from build123d import *

# Parameters (mm, degrees)
BOSS_EXTRU_1_DEPTH       = 68.5
BOSS_EXTRU_2_DEPTH       = 2.5
ESQUISSE4_W              = 95
ESQUISSE4_H              = 54.5
ENL_V_MAT_EXTRU_1_DEPTH  = 2.5
ESQUISSE5_W              = 16
ESQUISSE5_H              = 52.4
ENL_V_MAT_EXTRU_2_DEPTH  = 2.5
BOSS_EXTRU_3_DEPTH       = 2.5
CHANFREIN1_SIZE          = 2.5
CONG_1_R                 = 1.5
ENL_V_MAT_EXTRU_3_DEPTH  = 1.2
CHANFREIN2_SIZE          = 0.3
ESQUISSE8_W              = 20
ESQUISSE8_H              = 1
ENL_V_MAT_EXTRU_4_DEPTH  = 3
CHANFREIN3_SIZE          = 0.5
CHANFREIN4_SIZE          = 0.5
ESQUISSE9_R              = 1
ENL_V_MAT_EXTRU_5_DEPTH  = 75
CHANFREIN5_SIZE          = 1
CHANFREIN6_SIZE          = 1
ENL_V_MAT_EXTRU_6_DEPTH  = 1
ENL_V_START              = -1
ENL_V_MAT_EXTRU_7_DEPTH  = 1
ESQUISSE13_W             = 12
ESQUISSE13_H             = 8
ENL_V_MAT_EXTRU_8_DEPTH  = 2.5
CONG_2_R                 = 1
CHANFREIN7_SIZE          = 0.5
ESQUISSE14_W             = 25.2
ESQUISSE14_H             = 25.2
ENL_V_MAT_EXTRU_9_DEPTH  = 1.45
CHANFREIN8_SIZE          = 0.2
ESQUISSE15_R             = 10.1
ENL_V_MAT_EXTRU_10_DEPTH = 1.05
CHANFREIN9_SIZE          = 0.6


with BuildPart() as part:
    # Esquisse2 → Boss.-Extru.1 (new body)
    with BuildSketch(Plane(origin=(0, 0, 0), x_dir=(1, 0, 0), z_dir=(0, 1, 0))):
        Polygon((0, 0), (113, 0), (113, 40), (33, 40), (33, 38.7), (35.5, 38.7), (35.5, 37.5), (110.5, 37.5), (110.5, 2.5), (2.5, 2.5), (2.5, 1.3), (0, 1.3), align=None)
    extrude(amount=BOSS_EXTRU_1_DEPTH)

    # Esquisse3 → Boss.-Extru.2 (add)
    with BuildSketch(Plane.XZ):
        Polygon((0, 0), (113, 0), (113, -40), (33, -40), (33, -38.5), (0, -1.5), align=None)
    extrude(amount=BOSS_EXTRU_2_DEPTH)

    # Esquisse4 → Enlèv. mat.-Extru.1 (cut)
    with BuildSketch(Plane.XY):
        with Locations((57.3, 37.45)):
            Rectangle(ESQUISSE4_W, ESQUISSE4_H)
    extrude(amount=-ENL_V_MAT_EXTRU_1_DEPTH, mode=Mode.SUBTRACT)

    # Esquisse5 → Enlèv. mat.-Extru.2 (cut)
    with BuildSketch(Plane(origin=(113, 0, 0), x_dir=(0, 0, -1), z_dir=(1, 0, 0))):
        with Locations((24.8, 34.7)):
            Rectangle(ESQUISSE5_W, ESQUISSE5_H)
    extrude(amount=-ENL_V_MAT_EXTRU_2_DEPTH, mode=Mode.SUBTRACT)

    # Esquisse6 → Boss.-Extru.3 (add)
    with BuildSketch(Plane(origin=(0, 68.5, 0), x_dir=(1, 0, 0), z_dir=(0, 1, 0))):
        Polygon((33, 40), (33, 38.5), (0, 1.5), (0, 0), (113, 0), (113, 40), align=None)
    extrude(amount=BOSS_EXTRU_3_DEPTH)

    # Chanfrein1
    chanfrein1_edges = [part.edges().sort_by_distance(p)[0] for p in [
        (57.3, 10.2, 0),
        (104.8, 37.45, 0),
        (57.3, 64.7, 0),
        (9.8, 37.45, 0),
    ]]
    chamfer(chanfrein1_edges, length=CHANFREIN1_SIZE - 0.0001)  # a hair under: the kernel refuses the full size

    # Congé1
    cong_1_edges = [part.edges().sort_by_distance(p)[0] for p in [
        (73, -2.5, -40),
        (113, -2.5, -20),
        (113, 34.25, -40),
        (56.5, -2.5, 0),
        (113, 34.25, 0),
        (73, 71, -40),
        (113, 71, -20),
        (56.5, 71, 0),
    ]]
    fillet(cong_1_edges, radius=CONG_1_R)

    # Esquisse7 → Enlèv. mat.-Extru.3 (cut)
    with BuildSketch(Plane(origin=(0, 0, -40), x_dir=(-1, 0, 0), z_dir=(0, 0, -1))):
        Polygon((-86.45, 56.7), (-42.55, 56.7), (-42.55, 13.2), (-39.8, 13.2), (-39.8, 10.3), (-89.2, 10.3), (-89.2, 13.2), (-86.45, 13.2), align=None)
    extrude(amount=-ENL_V_MAT_EXTRU_3_DEPTH, mode=Mode.SUBTRACT)

    # Chanfrein2
    chanfrein2_edges = [part.edges().sort_by_distance(p)[0] for p in [
        (86.45, 34.95, -40),
        (87.825, 13.2, -40),
        (89.2, 11.75, -40),
        (64.5, 10.3, -40),
        (39.8, 11.75, -40),
        (41.175, 13.2, -40),
        (42.55, 34.95, -40),
        (64.5, 56.7, -40),
    ]]
    chamfer(chanfrein2_edges, length=CHANFREIN2_SIZE)

    # Esquisse8 → Enlèv. mat.-Extru.4 (cut)
    with BuildSketch(Plane(origin=(0, 0, -38.8), x_dir=(-1, 0, 0), z_dir=(0, 0, -1))):
        with Locations((-64.5, 56.2)):
            Rectangle(ESQUISSE8_W, ESQUISSE8_H)
    extrude(amount=-ENL_V_MAT_EXTRU_4_DEPTH, mode=Mode.SUBTRACT)

    # Chanfrein3
    chanfrein3_edges = [part.edges().sort_by_distance(p)[0] for p in [
        (74.5, 56.2, -38.8),
        (64.5, 55.7, -38.8),
        (54.5, 56.2, -38.8),
    ]]
    chamfer(chanfrein3_edges, length=CHANFREIN3_SIZE)

    # Chanfrein4
    chanfrein4_edges = [part.edges().sort_by_distance(p)[0] for p in [
        (64.5, 56.7, -37.5),
    ]]
    chamfer(chanfrein4_edges, length=CHANFREIN4_SIZE)

    # Esquisse9 → Enlèv. mat.-Extru.5 (cut)
    with BuildSketch(Plane(origin=(0, 71, 0), x_dir=(1, 0, 0), z_dir=(0, 1, 0))):
        with Locations(Location((20.92027027, 17.5, 0), (0, 0, 270))):
            Circle(ESQUISSE9_R)
        with Locations(Location((33.406756757, 31.5, 0), (0, 0, 270))):
            Circle(ESQUISSE9_R)
    extrude(amount=-ENL_V_MAT_EXTRU_5_DEPTH, mode=Mode.SUBTRACT)

    # Chanfrein5
    chanfrein5_edges = [part.edges().sort_by_distance(p)[0] for p in [
        (20.92027027, 71, -18.5),
        (33.406756757, 71, -32.5),
    ]]
    chamfer(chanfrein5_edges, length=CHANFREIN5_SIZE)

    # Chanfrein6
    chanfrein6_edges = [part.edges().sort_by_distance(p)[0] for p in [
        (20.92027027, -2.5, -18.5),
        (33.406756757, -2.5, -32.5),
    ]]
    chamfer(chanfrein6_edges, length=CHANFREIN6_SIZE)

    # Esquisse10 → Enlèv. mat.-Extru.6 (cut)
    with BuildSketch(Plane(origin=(0, 0, 0), x_dir=(1, 0, 0), z_dir=(0, 1, 0))):
        with BuildLine():
            Line((12.040050277, 15.299924377), (28.450890894, 33.699957797))
            Line((28.450890894, 33.699957797), (33.406738022, 33.7))
            ThreePointArc((33.406738022, 33.7), (35.606756752, 31.499854993), (33.406448008, 29.300000022))
            Line((33.406448008, 29.300000022), (28.735619265, 29.300655526))
            ThreePointArc((28.735619265, 29.300655526), (27.99947652, 29.143356281), (27.392034871, 28.698762269))
            Line((27.392034871, 28.698762269), (20.547584791, 21.024681875))
            ThreePointArc((20.547584791, 21.024681875), (20.399896986, 20.199981277), (21.069011886, 19.695770987))
            Line((21.069011886, 19.695770987), (21.128195715, 19.69015228))
            ThreePointArc((21.128195715, 19.69015228), (23.117807404, 17.395930099), (20.920289005, 15.3))
            Line((20.920289005, 15.3), (12.040050277, 15.299924377))
        make_face()
    extrude(amount=-ENL_V_MAT_EXTRU_6_DEPTH, mode=Mode.SUBTRACT)

    # Esquisse12 → Enlèv. mat.-Extru.7 (cut)
    with BuildSketch(Plane.XZ.offset(-68.5).offset(ENL_V_START)):
        with BuildLine():
            Line((12.308108108, -15.3), (20.92027027, -15.3))
            ThreePointArc((20.92027027, -15.3), (23.11421416, -17.336873648), (21.245624873, -19.675808903))
            Line((21.245624873, -19.675808903), (21.03224488, -19.707716192))
            ThreePointArc((21.03224488, -19.707716192), (20.398241002, -20.226848336), (20.553531675, -21.031425186))
            Line((20.553531675, -21.031425186), (27.392315335, -28.698793496))
            ThreePointArc((27.392315335, -28.698793496), (27.999748232, -29.143364838), (28.735871891, -29.300655526))
            Line((28.735871891, -29.300655526), (33.406447992, -29.300000022))
            ThreePointArc((33.406447992, -29.300000022), (35.606756752, -31.499854985), (33.406738022, -33.7))
            Line((33.406738022, -33.7), (28.718883313, -33.699960079))
            Line((28.718883313, -33.699960079), (12.308108108, -15.3))
        make_face()
    extrude(amount=ENL_V_MAT_EXTRU_7_DEPTH, mode=Mode.SUBTRACT)

    # Esquisse13 → Enlèv. mat.-Extru.8 (cut)
    with BuildSketch(Plane(origin=(0, 71, 0), x_dir=(1, 0, 0), z_dir=(0, 1, 0))):
        with Locations((34, 18.5)):
            Rectangle(ESQUISSE13_W, ESQUISSE13_H)
    extrude(amount=-ENL_V_MAT_EXTRU_8_DEPTH, mode=Mode.SUBTRACT)

    # Congé2
    cong_2_edges = [part.edges().sort_by_distance(p)[0] for p in [
        (28, 69.75, -14.5),
        (28, 69.75, -22.5),
        (40, 69.75, -22.5),
        (40, 69.75, -14.5),
    ]]
    fillet(cong_2_edges, radius=CONG_2_R)

    # Chanfrein7
    chanfrein7_edges = [part.edges().sort_by_distance(p)[0] for p in [
        (28, 71, -18.5),
        (34, 71, -22.5),
        (40, 71, -18.5),
        (34, 71, -14.5),
        (28.292893219, 71, -22.207106781),
        (39.707106781, 71, -22.207106781),
        (39.707106781, 71, -14.792893219),
        (28.292893219, 71, -14.792893219),
    ]]
    chamfer(chanfrein7_edges, length=CHANFREIN7_SIZE)

    # Esquisse14 → Enlèv. mat.-Extru.9 (cut)
    with BuildSketch(Plane(origin=(0, 71, 0), x_dir=(1, 0, 0), z_dir=(0, 1, 0))):
        with Locations((75.5, 20.5)):
            Rectangle(ESQUISSE14_W, ESQUISSE14_H)
    extrude(amount=-ENL_V_MAT_EXTRU_9_DEPTH, mode=Mode.SUBTRACT)

    # Chanfrein8
    chanfrein8_edges = [part.edges().sort_by_distance(p)[0] for p in [
        (62.9, 71, -20.5),
        (75.5, 71, -7.9),
        (88.1, 71, -20.5),
        (75.5, 71, -33.1),
    ]]
    chamfer(chanfrein8_edges, length=CHANFREIN8_SIZE)

    # Esquisse15 → Enlèv. mat.-Extru.10 (cut)
    with BuildSketch(Plane(origin=(0, 69.55, 0), x_dir=(1, 0, 0), z_dir=(0, 1, 0))):
        with Locations(Location((75.5, 20.5, 0), (0, 0, 270))):
            Circle(ESQUISSE15_R)
    extrude(amount=-ENL_V_MAT_EXTRU_10_DEPTH, mode=Mode.SUBTRACT)

    # Chanfrein9
    chanfrein9_edges = [part.edges().sort_by_distance(p)[0] for p in [
        (75.5, 69.55, -30.6),
    ]]
    chamfer(chanfrein9_edges, length=CHANFREIN9_SIZE)


solid = part.part
Verification items for the finished model (mm, model axes). A direction names the side the tool comes from. Coordinates: 2 decimals unless noted, no trailing zeros. One line per item, written item: value. Start each with the question number.
Item 1: Depth check by flat-ended pin: P1, Ø1.3, axis at y = 39, z = -2, coming from the -X side; P2, Ø0.8, axis at y = 20, z = -39.5, coming from the -X side; P3, Ø1.6, axis at y = 69, z = -18.5, coming from the -X side. Enter the tip coordinate at first touch or a pass-through.
Item 2: Thickness scan on probe 1 along Y at (x, z) = (40, -32.5); probe 2 along X at (y, z) = (68.6, -20.5); probe 3 along Z at (x, y) = (56, 2.5). Record the ranges inside material, lowest first.
Item 3: Sectioned sample at A-A on y = 27. Give the number of separate pieces and of enclosed holes in the cut face, then the cut area to 3 significant figures.
Item 4: Access from +Z, -Z, +X, -X, +Y, -Y to the whole of each face (thin tool, end or side, straight path). Record for faces 4 (the flat face through (1, 34, -1.3)), 5 (the flat face through (23, 69.5, -25)), 6 (the flat face through (112, 8.5, -25)), 7 (the flat face through (69, -2.5, -20)), 8 (the flat face through (75, 69.55, -9)).
Item 5: Mould release check, pull along X, two halves, no side actions. Record for faces 1 (the flat face through (113, 34, -16)), 2 (the flat face through (106.1, 37, -1.2)), 3 (the flat face through (68, 0, -20)): pulls with the +X half, pulls with the -X half, needs draft (parallel to the pull), parting line crosses it, or undercut.
Calculated:
1. P1: x = 2.5
1. P2: x = 33
1. P3: x = 14.61
2. probe 1: -2.5 to 0, 68.5 to 71
2. probe 2: 20.35 to 28, 40 to 65.4, 85.6 to 113
2. probe 3: -40 to -37.5, -2.5 to 0
3. separate pieces: 3
3. enclosed holes: 0
3. area: 227 mm^2
4. face 4: -Z, -X
4. face 5: -X
4. face 6: +X, -X
4. face 7: +Z, -Z, +X, -X, -Y
4. face 8: +Y
5. face 1: pulls with the +X half
5. face 2: undercut
5. face 3: needs draft
